Could you check a few things on this model? Use its own coordinates, in mm. Face numbers are marked on the shaded views. Give positions to 0.01 mm unless a question says otherwise; leave off trailing zeros. Loops run counter-clockwise (first coordinate to the right, second up) from the corner with the lowest first, then second, coordinate; pieces in that order, holes last. Notation, with made-up numbers: (40, 73.5) - (74, 73.5) arc R20 cw to (74, 88.5) - close; hole circle Ø5 at (16, 30.5). An arc over 180 degrees is marked (long way). Answer in a Markdown table with one row per item. Add a question column.
```python
from build123d import *

# Parameters (mm, degrees)
CYLINDER005_R     = 1.4
CYLINDER005_DEPTH = 10
EXTRUDE001_DEPTH  = 2
SKETCH002_R       = 1.4
EXTRUDE002_DEPTH  = 6
EXTRUDE_DEPTH     = 1


with BuildPart() as cylinder005:
    # Cylinder005 → Cylinder005 (new body)
    with BuildSketch(Plane(origin=(-5, 2.5, -5), x_dir=(1, 0, 0), z_dir=(0, 0, 1))):
        Circle(CYLINDER005_R)
    extrude(amount=CYLINDER005_DEPTH)


with BuildPart() as extrude001:
    # Sketch001 → Extrude001 (new body)
    with BuildSketch(Plane.XY.offset(10)):
        Polygon((-21, 10), (0, 10), (0, 9), (-20, 9), (-20, 1), (0, 1), (0, 0), (-21, 0), align=None)
        Polygon((-21, -1.5), (-12.25, -1.5), (-12.25, -21.5), (-13.25, -21.5), (-13.25, -2.5), (-20, -2.5), (-20, -21.5), (-21, -21.5), align=None)
    extrude(amount=-EXTRUDE001_DEPTH)


with BuildPart() as extrude001_1:
    # Extrude001 placement: moved
    add(extrude001.part.moved(Location((0, 0, -8))))


with BuildPart() as extrude002:
    # Sketch002 → Extrude002 (new body)
    with BuildSketch(Plane.XY.offset(10)):
        with BuildLine():
            ThreePointArc((-2.695656, 0), (-5, 5.9), (-7.304344, 0))
            Line((-7.304344, 0), (-2.695656, 0))
        make_face()
        with Locations((-5, 2.5)):
            Circle(SKETCH002_R, mode=Mode.SUBTRACT)
    extrude(amount=-EXTRUDE002_DEPTH)


with BuildPart() as extrude002_1:
    # Extrude002 placement: moved
    add(extrude002.part.moved(Location((0, 0, -7))))


with BuildPart() as body002:
    # Sketch → Extrude (new body)
    with BuildSketch(Plane.XY):
        Polygon((-11, 0), (0, 0), (0, 10), (-21, 10), (-21, -21.5), (-11, -21.5), align=None)
    extrude(amount=EXTRUDE_DEPTH)


with BuildPart() as body002_1:
    # Extrude placement: moved
    add(body002.part.moved(Location((0, 0, 2))))

    # Fusion012: union Extrude001, Extrude002
    add(extrude001_1.part)
    add(extrude002_1.part)

    # Cut001: cut Cylinder005
    add(cylinder005.part, mode=Mode.SUBTRACT)


with BuildPart() as part_mirroring003:
    # Part__Mirroring003: instance of Body002
    add(body002_1.part.mirror(Plane(origin=(0, 0, 0), x_dir=(0, -1, 0), z_dir=(1, 0, 0))))


solid = part_mirroring003.part
```
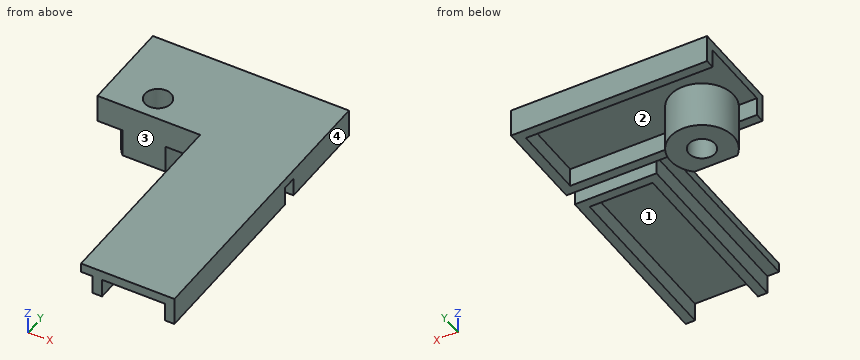
(1) I want a section at C-C on y = -4.5. Please give me the cut outline in (x, z), then the cut area to 3 significant figures.
(2) We'd pull the mould along X, two halves only. Please class the marked faces 1, 2, 3 and 4: pulls with the +X half, pulls with the -X half, needs draft (parallel to the pull), parting line crosses it, or undercut.
(3) I want a section at B-B on x = 5. Please give me the cut outline in (y, z), then the cut area to 3 significant figures.
(4) For pin 1 Ø3 at (x, z) = (8, 1.5) entering from -Y; pin 2 Ø3.5 at (x, y) = (17, -14.5) entering from -Z; pin 3 Ø0.8 at (y, z) = (-6, 2.5) entering from -X, each with a flat end and sliding along its axis, tell me the tip position at first contact or that it passes through.
(5) I want a section at D-D on x = 15.25. Please give me the cut outline in (y, z).
(6) Please list where these lines run through material, in increasing order: line 1 (Y direction, x = 19.25, z = 1.85); line 2 (X direction, y = 2.5, z = 0.65); line 3 (Y direction, x = 4, z = 0.1).
(7) I want a section at A-A on y = 2.5. Please give me the cut outline in (x, z), then the cut area to 3 significant figures.
Reported:
| question | item | result |
|---|---|---|
| 1 | outline | (11, 2) - (12.25, 2) - (12.25, 0) - (13.25, 0) - (13.25, 2) - (20, 2) - (20, 0) - (21, 0) - (21, 3) - (11, 3) - close |
| 1 | area | 14.0 mm² |
| 2 | face 1 | undercut |
| 2 | face 2 | undercut |
| 2 | face 3 | needs draft |
| 2 | face 4 | pulls with the +X half |
| 3 | outline | (0, -3) - (1.1, -3) - (1.1, 3) - (0, 3) - close; (3.9, -3) - (5.9, -3) - (5.9, 2) - (9, 2) - (9, 0) - (10, 0) - (10, 3) - (3.9, 3) - close |
| 3 | area | 24.7 mm² |
| 4 | pin 1 | y = 0 |
| 4 | pin 2 | z = 2 |
| 4 | pin 3 | x = 11 |
| 5 | outline | (-21.5, 2) - (-2.5, 2) - (-2.5, 0) - (-1.5, 0) - (-1.5, 2) - (0, 2) - (0, 0) - (1, 0) - (1, 2) - (9, 2) - (9, 0) - (10, 0) - (10, 3) - (-21.5, 3) - close |
| 6 | line 1 | -2.5 to -1.5, 0 to 1, 9 to 10 |
| 6 | line 2 | 1.6 to 3.6, 6.4 to 8.4, 20 to 21 |
| 6 | line 3 | 0 to 1.52, 3.48 to 5.75, 9 to 10 |
| 7 | outline | (0, 2) - (1.6, 2) - (1.6, -3) - (3.6, -3) - (3.6, 3) - (0, 3) - close; (6.4, -3) - (8.4, -3) - (8.4, 2) - (20, 2) - (20, 0) - (21, 0) - (21, 3) - (6.4, 3) - close |
| 7 | area | 40.2 mm² |
